```python
from build123d import *

# Parameters (mm, degrees)
SKETCH1_R           = 2
BOSS_EXTRUDE1_DEPTH = 6
SCALE1_SCALE        = 7.5


with BuildPart() as part:
    # Sketch1 → Boss-Extrude1 (new body)
    with BuildSketch(Plane(origin=(0, 0, 0), x_dir=(1, 0, 0), z_dir=(0, 1, 0))):
        with BuildLine():
            Line((-27, -27), (-27, -47))
            ThreePointArc((-27, -47), (-24.071067812, -54.071067812), (-17, -57))
            Line((-17, -57), (43, -57))
            ThreePointArc((43, -57), (50.071067812, -54.071067812), (53, -47))
            Line((53, -47), (53, -27))
            Line((53, -27), (53, 93))
            ThreePointArc((53, 93), (50.071067812, 100.071067812), (43, 103))
            Line((43, 103), (-17, 103))
            ThreePointArc((-17, 103), (-24.071067812, 100.071067812), (-27, 93))
            Line((-27, 93), (-27, -27))
        make_face()
        with Locations((13, 89.666666667)):
            Circle(SKETCH1_R, mode=Mode.SUBTRACT)
        with Locations((13, 49.666666667)):
            Circle(SKETCH1_R, mode=Mode.SUBTRACT)
        with Locations((13, 9.666666667)):
            Circle(SKETCH1_R, mode=Mode.SUBTRACT)
        with Locations((13, -30.333333333)):
            Circle(SKETCH1_R, mode=Mode.SUBTRACT)
    extrude(amount=BOSS_EXTRUDE1_DEPTH)


with BuildPart() as part_1:
    # Scale1: scaled about (13, 3, -22.97353869)
    add(part.part.scale(SCALE1_SCALE).moved(Location((-84.5, -19.5, 149.328001485))))


solid = part_1.part
```
CAD build for the part. Positions are in the model's coordinates, mm. Round coordinates to 2 decimals unless told otherwise and drop trailing zeros. Order: outer loops, then holes, each group sorted by start corner. A loop starts at its lowest first (then second) coordinate and runs counter-clockwise, first axis right, second up. Notation, with made-up numbers: (23.25, 42.25) -> (57.25, 42.25) arc R17 ccw to (57.25, 67.25) -> close; hole circle Ø10 at (6.25, -36). An arc over 180 degrees is marked (long way). Write item = value, one per line.
(1) Pull direction Z, two halves, no side cores. Call faces 1 (the flat face through (9, 25.5, -32)), 2 (the flat face through (16, 3, -623.172)), 3 (the cylindrical face through (9.75, 2.68, -508.53)): +Z half, -Z half, draft (parallel to the pull), parting line (faces both ways), or undercut.
Answers follow:
face_1 = draft
face_2 = -Z half
face_3 = undercut
(2) Cut at A-A (x = 13). Write the cut outline in (y, z), plus the area to 3 significant figures.
Answers follow:
outline = (-19.5, -623.17) -> (25.5, -623.17) -> (25.5, -538.17) -> (-19.5, -538.17) -> close; (-19.5, -508.17) -> (25.5, -508.17) -> (25.5, -238.17) -> (-19.5, -238.17) -> close; (-19.5, -208.17) -> (25.5, -208.17) -> (25.5, 61.83) -> (-19.5, 61.83) -> close; (-19.5, 91.83) -> (25.5, 91.83) -> (25.5, 361.83) -> (-19.5, 361.83) -> close; (-19.5, 391.83) -> (25.5, 391.83) -> (25.5, 576.83) -> (-19.5, 576.83) -> close
area = 48,600 mm²
(3) Drill centre lines: L1, parallel to Z at x = 13, y = 0; L2, parallel to X at y = -0.5, z = 79; L3, parallel to X at y = 3, z = -566. Where is each one in solid material? Low to high.
Answers follow:
L1 = -623.17 to -538.17, -508.17 to -238.17, -208.17 to 61.83, 91.83 to 361.83, 391.83 to 576.83
L2 = -287 to -1.84, 27.84 to 313
L3 = -284.85 to 310.85
(4) Flat gauge pin, fed straight in: P1, Ø24, axis at x = 13, z = 376.83, coming from the -Y side. Where does the tip first touch, or does it go through?
Answers follow:
P1 = through
